CAD build for the part. Positions are in the model's coordinates, mm. Coordinates: 2 decimals unless noted, no trailing zeros. Order: outer loops, then holes, each group sorted by start corner. A loop starts at its lowest first (then second) coordinate and runs counter-clockwise, first axis right, second up. Notation, with made-up numbers: (74, 52.25) - (97, 52.25) arc R11 cw to (97, 70.25) - close; hole circle Ø9 at (8, 25). An arc over 180 degrees is marked (long way). Use one line per item in the form item = value.
```python
from build123d import *

# Parameters (mm, degrees)
EXTRUDE_1_DEPTH = 4
CHAMFER_1_SIZE  = 0.5


with BuildPart() as part:
    # 草图1 → 凸台-拉伸1 (new body)
    with BuildSketch(Plane(origin=(0, 0, 0), x_dir=(1, 0, 0), z_dir=(0, 1, 0))):
        with BuildLine():
            Line((-8.5, -1.5), (8.5, -1.5))
            ThreePointArc((8.5, -1.5), (10, 0), (8.5, 1.5))
            Line((8.5, 1.5), (-8.5, 1.5))
            ThreePointArc((-8.5, 1.5), (-10, 0), (-8.5, -1.5))
        make_face()
    extrude(amount=EXTRUDE_1_DEPTH)

    # 倒角1
    chamfer_1_edges = [part.edges().sort_by_distance(p)[0] for p in [
        (0, 0, 1.5),
        (-10, 0, 0),
        (0, 0, -1.5),
        (10, 0, 0),
    ]]
    chamfer(chamfer_1_edges, length=CHAMFER_1_SIZE)


solid = part.part
```
Item 1: Cut at A-A, the plane x = 4.25. Write the cut outline in (y, z).
Derived:
outline = (0, -1) - (0.5, -1.5) - (4, -1.5) - (4, 1.5) - (0.5, 1.5) - (0, 1) - close
Item 2: Drill centre lines: line 1 (X direction, y = 2.65, z = -0.1); line 2 (X direction, y = 1.75, z = -0.5); line 3 (Y direction, x = -8.5, z = -1.35). Where is each one in solid material? Low to high. Write a range as [from, to].
Derived:
line_1 = [-10, 10]
line_2 = [-9.91, 9.91]
line_3 = [0.35, 4]
Item 3: Drop a flat-ended pin along its axis: pin 1 (1.5 mm diameter, centred on y = 2.5, z = 1, fed in from -X). Give the stop position or say it passes through.
Derived:
pin_1 = -9.98
Item 4: Cut at B-B, the plane y = 0.8. Write the cut outline in (x, z).
Derived:
outline = (-8.5, -1.5) - (8.5, -1.5) arc R1.5 ccw to (8.5, 1.5) - (-8.5, 1.5) arc R1.5 ccw to start
